Check sheet for the modelled part. Datum: model origin and axes. Units: mm. Face numbers are marked on the shaded views. A direction names the side the tool comes from. Round coordinates to 2 decimals unless told otherwise and drop trailing zeros. Order: outer loops, then holes, each group sorted by start corner. A loop starts at its lowest first (then second) coordinate and runs counter-clockwise, first axis right, second up. Notation, with made-up numbers: (58.5, -30) -> (77.5, -30) arc R18 ccw to (77.5, -24) -> close; hole circle Ø5 at (78.5, 31). An arc over 180 degrees is marked (long way). Use CSV: the item, a comma, the result in double quotes.
```python
from build123d import *

# Parameters (mm, degrees)
CROQUIS1_W                   = 75.5
CROQUIS1_H                   = 40.8
SALIENTE_EXTRUIR1_DEPTH      = 16
VACIADO1_T                   = -1.8
SALIENTE_EXTRUIR2_DEPTH      = 0.3
SALIENTE_EXTRUIR2_DEPTH_BACK = 0.3
CROQUIS2_W                   = 71.9
CROQUIS2_H                   = 9
CORTAR_EXTRUIR1_REACH        = 81.827
CROQUIS3_R                   = 1.25
MATRIZL1_COUNT               = 2
MATRIZL1_PITCH               = 18.8
REDONDEO1_R                  = 2


with BuildPart() as part:
    # Croquis1 → Saliente-Extruir1 (new body)
    with BuildSketch(Plane(origin=(0, 0, 0), x_dir=(1, 0, 0), z_dir=(0, 1, 0))):
        Rectangle(CROQUIS1_W, CROQUIS1_H)
    extrude(amount=SALIENTE_EXTRUIR1_DEPTH)

    # Vaciado1
    vaciado1_openings = [part.faces().sort_by_distance(p)[0] for p in [
        (0, 16, 0),
    ]]
    offset(amount=VACIADO1_T, openings=vaciado1_openings, kind=Kind.INTERSECTION)

    # Croquis2 → Saliente-Extruir2 (add, two sides: drawn at the far end of the back side and taken through both)
    with BuildSketch(Plane.XY.offset(-SALIENTE_EXTRUIR2_DEPTH_BACK)):
        with Locations((0, 6.3)):
            Rectangle(CROQUIS2_W, CROQUIS2_H)
    extrude(amount=SALIENTE_EXTRUIR2_DEPTH + SALIENTE_EXTRUIR2_DEPTH_BACK)

    # Cortar-Extruir1: up to this face of the body (flat: up to its plane)
    cortar_extruir1_end = Plane(part.part.faces().sort_by_distance((37.75, 8, 0))[0])
    # Croquis3 → Cortar-Extruir1 (cut, up to the picked face)
    with BuildSketch(Plane.ZY.offset(37.75), mode=Mode.PRIVATE) as cortar_extruir1_sk1:
        with Locations((9.4, 9.1)):
            Circle(CROQUIS3_R)
    cortar_extruir1_tool1 = split(extrude(cortar_extruir1_sk1.sketch, amount=-CORTAR_EXTRUIR1_REACH, mode=Mode.PRIVATE), bisect_by=cortar_extruir1_end, keep=Keep.BOTH, mode=Mode.PRIVATE)
    cortar_extruir1 = cortar_extruir1_tool1.solids().sort_by(Axis((-37.75, 9.1, 9.4), (1, 0, 0)))[0]
    add(cortar_extruir1, mode=Mode.SUBTRACT)

    # MatrizL1: Cortar-Extruir1 ×2
    with Locations(*[(0, 0, -i * MATRIZL1_PITCH) for i in range(1, MATRIZL1_COUNT)]):
        add(cortar_extruir1, mode=Mode.SUBTRACT)

    # Redondeo1
    # the kernel refuses this fillet: 2 mm, written as the material it takes off along each edge
    with BuildSketch(Plane(origin=(-42.75, 16, -20.4), x_dir=(0, -1, 0), z_dir=(1, 0, 0))) as redondeo1_piece_1:
        with BuildLine():
            CenterArc((REDONDEO1_R, -REDONDEO1_R), REDONDEO1_R, 90, 90)
            Line((0, -REDONDEO1_R), (0, 0))
            Line((0, 0), (REDONDEO1_R, 0))
        make_face()
    extrude(amount=85.5, mode=Mode.SUBTRACT)
    with BuildSketch(Plane(origin=(-37.75, 16, 25.4), x_dir=(0, -1, 0), z_dir=(0, 0, -1)), Plane(origin=(37.75, 16, -25.4), x_dir=(0, -1, 0), z_dir=(0, 0, 1))) as redondeo1_piece_2:
        with BuildLine():
            CenterArc((REDONDEO1_R, -REDONDEO1_R), REDONDEO1_R, 90, 90)
            Line((0, -REDONDEO1_R), (0, 0))
            Line((0, 0), (REDONDEO1_R, 0))
        make_face()
    extrude(amount=50.8, mode=Mode.SUBTRACT)
    with BuildSketch(Plane(origin=(42.75, 16, 20.4), x_dir=(0, 0, -1), z_dir=(-1, 0, 0))) as redondeo1_piece_3:
        with BuildLine():
            CenterArc((REDONDEO1_R, REDONDEO1_R), REDONDEO1_R, 180, 90)
            Line((0, REDONDEO1_R), (0, 0))
            Line((0, 0), (REDONDEO1_R, 0))
        make_face()
    extrude(amount=85.5, mode=Mode.SUBTRACT)


solid = part.part
```
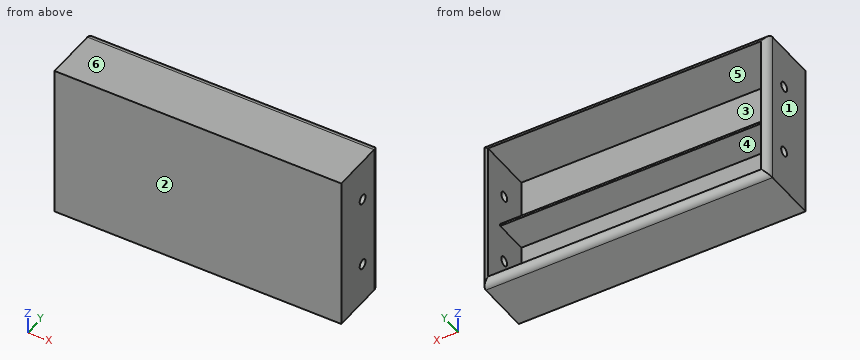
Q1. Go/stop test with flat-tipped pins: pin 1 (0.5 mm diameter, centred on x = 11.5, z = 0, fed in from +Y); pin 2 (5.5 mm diameter, centred on x = 3, z = -11, fed in from +Y). Record where each tip stops, or that it passes through.
Result sheet:
pin 1,"stops at y = 10.8"
pin 2,"stops at y = 1.8"
Q2. Sectioned sample at B-B, the plane z = 1. Enter the section's corners in (x, y).
Result sheet:
outline,"(-37.75, 0) -> (37.75, 0) -> (37.75, 14) arc R2 ccw to (35.95, 15.99) -> (35.95, 1.8) -> (-35.95, 1.8) -> (-35.95, 15.99) arc R2 ccw to (-37.75, 14) -> close"
Q3. Access from +Z, -Z, +X, -X, +Y, -Y to the whole of each face (thin tool, end or side, straight path). Record for the marked faces 5 and 6.
Result sheet:
face 5,"+Y"
face 6,"+Z, +X, -X, +Y, -Y"
Q4. Mould release check, pull along X, two halves, no side actions. Record for the marked faces 1, 2, 3 and 4: pulls with the +X half, pulls with the -X half, needs draft (parallel to the pull), parting line crosses it, or undercut.
Result sheet:
face 1,"pulls with the -X half"
face 2,"needs draft"
face 3,"undercut"
face 4,"undercut"
Q5. Sectioned sample at C-C, the plane x = -5.5. Enter the section's corners in (y, z).
Result sheet:
outline,"(0, -20.4) -> (14, -20.4) arc R2 ccw to (15.99, -18.6) -> (1.8, -18.6) -> (1.8, -0.3) -> (10.8, -0.3) -> (10.8, 0.3) -> (1.8, 0.3) -> (1.8, 18.6) -> (15.99, 18.6) arc R2 ccw to (14, 20.4) -> (0, 20.4) -> close"
Q6. Sectioned sample at D-D, the plane z = 9.4. Enter the section's corners in (x, y), then the cut area to 3 significant figures.
Result sheet:
outline,"(-37.75, 0) -> (37.75, 0) -> (37.75, 7.85) -> (35.95, 7.85) -> (35.95, 1.8) -> (-35.95, 1.8) -> (-35.95, 7.85) -> (-37.75, 7.85) -> close; (-37.75, 10.35) -> (-35.95, 10.35) -> (-35.95, 15.99) arc R2 ccw to (-37.75, 14) -> close; (35.95, 10.35) -> (37.75, 10.35) -> (37.75, 14) arc R2 ccw to (35.95, 15.99) -> close"
area,"176 mm^2"
Q7. Sectioned sample at A-A, the plane y = 9.1. Enter the section's corners in (x, z).
Result sheet:
outline,"(-37.75, -20.4) -> (37.75, -20.4) -> (37.75, -10.65) -> (35.95, -10.65) -> (35.95, -18.6) -> (-35.95, -18.6) -> (-35.95, -10.65) -> (-37.75, -10.65) -> close; (-37.75, -8.15) -> (-35.95, -8.15) -> (-35.95, -0.3) -> (35.95, -0.3) -> (35.95, -8.15) -> (37.75, -8.15) -> (37.75, 8.15) -> (35.95, 8.15) -> (35.95, 0.3) -> (-35.95, 0.3) -> (-35.95, 8.15) -> (-37.75, 8.15) -> close; (-37.75, 10.65) -> (-35.95, 10.65) -> (-35.95, 18.6) -> (35.95, 18.6) -> (35.95, 10.65) -> (37.75, 10.65) -> (37.75, 20.4) -> (-37.75, 20.4) -> close"
Q8. Scan lines: L1, parallel to Z at x = -6.5, y = 2.5; L2, parallel to X at y = 9.5, z = -17.5; L3, parallel to Z at x = 17.5, y = 14.25. Record each from-to range of solid material in increasing order.
Result sheet:
L1,"z = -20.4 to -18.6, -0.3 to 0.3, 18.6 to 20.4"
L2,"x = -37.75 to -35.95, 35.95 to 37.75"
L3,"z = -20.38 to -18.6, 18.6 to 20.38"
